Check sheet for the modelled part. Datum: model origin and axes. Units: mm. A direction names the side the tool comes from. Give positions to 0.01 mm unless a question says otherwise; leave off trailing zeros. Write each loop counter-clockwise with the first axis right and the second up, starting at its lowest first coordinate (ties: lowest second). Pieces come first, ordered by that corner, then holes. Notation, with made-up numbers: (34, 43) -> (61, 43) arc R23 ccw to (61, 61) -> close; hole circle Ø6 at (-11, 69). An arc over 180 degrees is marked (long way). Answer as a JSON object with one key per item and string values.
from build123d import *

# Parameters (mm, degrees)
SKETCH1_W           = 30
SKETCH1_H           = 30
BOSS_EXTRUDE1_DEPTH = 26
SHELL1_T            = -3
SKETCH3_R           = 4
CUT_EXTRUDE1_DEPTH  = 43.438190348
BOSS_EXTRUDE2_REACH = 50.497
SKETCH6_W           = 30
SKETCH6_H           = 30


with BuildPart() as part:
    # Sketch1 → Boss-Extrude1 (new body)
    with BuildSketch(Plane(origin=(0, 0, 0), x_dir=(1, 0, 0), z_dir=(0, 1, 0))):
        Rectangle(SKETCH1_W, SKETCH1_H)
    extrude(amount=BOSS_EXTRUDE1_DEPTH)

    # Shell1
    shell1_openings = [part.faces().sort_by_distance(p)[0] for p in [
        (-15, 13, 0),
        (15, 13, 0),
    ]]
    offset(amount=SHELL1_T, openings=shell1_openings, kind=Kind.INTERSECTION)

    # Sketch3 → Cut-Extrude1 (cut, through all)
    with BuildSketch(Plane.XY.offset(15)):
        with Locations((0, 13)):
            Circle(SKETCH3_R)
    extrude(amount=-CUT_EXTRUDE1_DEPTH, mode=Mode.SUBTRACT)


with BuildPart() as body_2:
    # Sketch5 → Revolve1 (revolve)
    with BuildSketch(Plane.XY):
        with BuildLine():
            Line((-28, 54), (-26, 54))
            ThreePointArc((-26, 54), (-18.384776311, 35.615223689), (0, 28))
            Line((0, 28), (0, 26))
            ThreePointArc((0, 26), (-19.798989873, 34.201010127), (-28, 54))
        make_face()
    revolve(axis=Axis((0, 26, 0), (0, 1, 0)))

    # Sketch6 → Boss-Extrude2 (add, up to next)
    with BuildSketch(Plane(origin=(0, 26, 0), x_dir=(1, 0, 0), z_dir=(0, 1, 0)), mode=Mode.PRIVATE) as boss_extrude2_sk1:
        Rectangle(SKETCH6_W, SKETCH6_H)
    boss_extrude2_tool1 = extrude(boss_extrude2_sk1.sketch, amount=BOSS_EXTRUDE2_REACH, mode=Mode.PRIVATE) - body_2.part

    add(part.part)  # Boss-Extrude2 merges part
    add(boss_extrude2_tool1.solids().sort_by_distance((0, 26, 0))[0])


solid = body_2.part
1. Sectioned sample at C-C, the plane z = 6.5. Enter the section's corners in (x, y).
Determined:
{"outline": "(-27.24, 54) arc R27.24 ccw to (-15, 31.27) -> (-15, 23) -> (15, 23) -> (15, 31.27) arc R27.24 ccw to (27.24, 54) -> (25.17, 54) arc R25.17 cw to (-25.17, 54) -> close; (-15, 0) -> (15, 0) -> (15, 3) -> (-15, 3) -> close"}
2. Go/stop test with flat-tipped pins: P1, Ø5, axis at x = 9, y = 47.5, coming from the -Z side; P2, Ø6, axis at x = 1.5, y = 8, coming from the -Z side; P3, Ø7, axis at x = -6, z = 0.5, coming from the +Y side; P4, Ø5, axis at x = 0, y = 13, coming from the -Z side. Record where each tip stops, or that it passes through.
Determined:
{"P1": "z = -26.65", "P2": "z = -15", "P3": "y = 29.81", "P4": "through"}
3. Access from +Z, -Z, +X, -X, +Y, -Y to the whole of each face (thin tool, end or side, straight path). Record for faces 1 (the face through (-0.521, 16.966, 13.521)), 2 (the face through (-4, 15, -12)).
Determined:
{"face 1": "+Z, -Z", "face 2": "+X, -X"}
4. Scan lines: L1, parallel to Z at x = 22, y = 47; L2, parallel to Z at x = 6.5, y = 37; L3, parallel to Z at x = 5, y = 27. Record each from-to range of solid material in increasing order. Write a range as [from, to].
Determined:
{"L1": "[-15.84, -11.96], [11.96, 15.84]", "L2": "[-21.28, -18.57], [18.57, 21.28]", "L3": "[-15, 15]"}
5. Mould release check, pull along Z, two halves, no side actions. Record for faces 3 (the face through (-4, 15, 12)), 4 (the face through (-0.521, 16.966, -13.479)), 5 (the face through (0, 18, 15)): released by +Z, released by -Z, zero draft, split by the parting line, or undercut.
Determined:
{"face 3": "undercut", "face 4": "zero draft", "face 5": "released by +Z"}
6. Sectioned sample at D-D, the plane x = 6. Enter the section's corners in (y, z), plus the area to 3 significant figures.
Determined:
{"outline": "(0, -15) -> (31.13, -15) arc R27.35 ccw to (54, -27.35) -> (54, -25.3) arc R25.3 cw to (54, 25.3) -> (54, 27.35) arc R27.35 ccw to (31.13, 15) -> (0, 15) -> close; hole (3, -12) -> (23, -12) -> (23, 12) -> (3, 12) -> close", "area": "532 mm^2"}
7. Sectioned sample at B-B, the plane y = 13. Enter the section's corners in (x, z).
Determined:
{"outline": "(-15, -15) -> (-4, -15) -> (-4, -12) -> (-15, -12) -> close; (-15, 12) -> (-4, 12) -> (-4, 15) -> (-15, 15) -> close; (4, -15) -> (15, -15) -> (15, -12) -> (4, -12) -> close; (4, 12) -> (15, 12) -> (15, 15) -> (4, 15) -> close"}
8. Sectioned sample at A-A, the plane x = 0. Enter the section's corners in (y, z).
Determined:
{"outline": "(0, -15) -> (9, -15) -> (9, -12) -> (3, -12) -> (3, 12) -> (9, 12) -> (9, 15) -> (0, 15) -> close; (17, -15) -> (30.36, -15) arc R28 ccw to (54, -28) -> (54, -26) arc R26 cw to (54, 26) -> (54, 28) arc R28 ccw to (30.36, 15) -> (17, 15) -> (17, 12) -> (23, 12) -> (23, -12) -> (17, -12) -> close"}
